Input: part model. Units: mm. Frame: model coordinates. Face numbers are marked on the shaded views. A direction names the side the tool comes from. Give positions to 0.01 mm unless a question says otherwise; leave off trailing zeros. Loops run counter-clockwise (first coordinate to the right, second up) from the corner with the lowest first, then second, coordinate; pieces in that order, holes last. Notation, with made-up numbers: M 52,-1.5 L 71,-1.5 A8 cw 71,5.5 Z; hole C 65,61.5 d11. An arc over 180 degrees is marked long. Answer as a JSON object with one key per item and string values. Group by question number.
1) First-contact query: P1, Ø2, axis at x = 0, z = -1.5, coming from the +Y side; P2, Ø1, axis at y = -3, z = -2.5, coming from the +X side; P3, Ø4, axis at x = 5.5, y = -1.5, coming from the -Z side. Flat tips, straight axial feed; report the tip coordinate or a pass-through.
2) Section query B-B on x = 6.75. Return loops of the section in (y, z), plus the area to 3 significant figures.
3) Ray query, L1, parallel to Y at x = 14, z = 1.5; L2, parallel to X at y = -3.25, z = 0.25; L3, parallel to X at y = 3, z = -2.25. Return the intervals inside material, ascending.
4) Access query for the marked faces 1 and 2. Directions: +Z, -Z, +X, -X, +Y, -Y. A direction counts if a zero-diameter tool reaches every point of the face in a straight line with its end or side. Return the directions, or none.
5) Section query A-A on x = -1. Return loops of the section in (y, z).
Autodesk Inventor part; units mm, degrees
ref_plane "Work Plane1" through (1.525, 0, 0) normal (0, 0, 1) x (1, 0, 0)
ref_plane "YZ Plane" through (0, 0, 0) normal (1, 0, 0) x (0, 1, 0)
ref_plane "XZ Plane" through (0, 0, 0) normal (0, 1, 0) x (-1, 0, 0)
sketch "Sketch1" plane through (0, 0, 0) normal (0, 0, 1) x (1, 0, 0)
  line L0 (0, 3.44) -> (0, 2.5)
  line L1 (2.4, 2.5) -> (20, 2.5)
  line L2 (20, 2.5) -> (20, 0)
  line L3 (20, 0) -> (-0.5001, 0)
  line L4 (-4.6001, 0) -> (24.1, 0)
  line L5 (-0.5001, 0) -> (-0.5001, 3.44)
  line L6 (-0.5001, 3.44) -> (0, 3.44)
  line L7 (2.4, 2.5) -> (1.9091, 2.5)
  line L8 (1.9091, 2.5) -> (0, 2.5)
  line L9 (0, -0.688) -> (0, 4.128)
  dimension "d0" = 20
  dimension "d1" = 17.6
  dimension "d2" = 5
  dimension "d9" = 0.5001
  dimension "d10" = 6.88
  dimension "d13" = 0.4909
  dimension "d14" = 5
revolve "Body" add sketch "Sketch1" angle 360 about axis through (20, 0, 0) along (-1, 0, 0)
sketch "Sketch2" plane through (-0.5001, 0, 0) normal (-1, 0, 0) x (0, 0, 1)
  line L0 (0, 4.6188) -> (4, 2.3094)
  line L1 (4, 2.3094) -> (4, -2.3094)
  line L2 (4, -2.3094) -> (0, -4.6188)
  line L3 (0, -4.6188) -> (-4, -2.3094)
  line L4 (-4, -2.3094) -> (-4, 2.3094)
  line L5 (-4, 2.3094) -> (0, 4.6188)
  point P0 (0, 0)
  point P1 (0, 0)
  dimension "d11" = 8
extrude "Head" add sketch "Sketch2" along normal blind 3
sketch "Sketch4" plane through (0, 0, 0) normal (0, 0, 1) x (1, 0, 0)
  line L0 (-3.5001, 4) -> (-3.5001, 4.6188)
  line L1 (-3.5001, 4.6188) -> (-3.1428, 4.6188)
  line L2 (-3.1428, 4.6188) -> (-3.5001, 4)
  line L3 (-4.1001, 0) -> (0.0999, 0)
  line L4 (-0.5001, 4.6188) -> (-3.5001, 4.6188)
  line L5 (-3.5001, 2.3094) -> (-3.5001, 4.6188)
  dimension "d5" = 30
  dimension "d19" = 8
revolve "Chamfer1" cut sketch "Sketch4" angle 360 about axis through (-10, 0, 0) along (1, 0, 0)
thread "Thread"
chamfer "Chamfer2" distance 0.4908 distance2 0.4909 1 edges at (20, -2.5, 0) measured on face at (20, 0.7379, -0.3873)
ref_plane "Work Plane1" through (1.525, 0, 0) normal (0, 0, 1) x (1, 0, 0)
equation "\"d0\" = NLG"
equation "\"d1\" = GEL"
equation "\"d2\" = GD"
equation "\"d10\" = SD2"
equation "\"d14\" = BDM"
equation "\"d11\" = SW"
equation "\"d3\" = KOH - SD"
equation "\"d5\" = ANG1"
equation "\"d19\" = SW0"
equation "\"d15\" = GEL"
equation "\"d6\" = -0.5 * SPD + 0.5 * GD"
equation "\"NLG\" = 20"
equation "\"GD\" = NND"
equation "\"BDM\" = NND"
equation "\"KOH\" = 3.5"
equation "\"GEL\" = 17.6"
equation "\"SW\" = 8"
equation "\"SW0\" = SW"
equation "\"SPD\" = NND - 1.2269 * PTC"
equation "\"SD2\" = 6.88"
equation "\"SD\" = 0.5"
equation "\"ANG1\" = 30deg"
equation "\"GAL\" = 0.61345 * PTC"
equation "\"GUL\" = 0.61345 * PTC"
equation "\"RR\" = 0.2"
equation "\"GD1\" = THREADDIA - 1.2269 * PTC"
equation "\"THREADDIA\" = 5"
equation "\"SDH\" = SD2"
equation "\"SDHG\" = 2.4"
equation "\"TOA\" = 30deg"
equation "\"PTC\" = 0.8"
equation "\"NND\" = 5"
equation "\"E0\" = 9.24"
properties part number "ISO 4017 - M5 x 20" material "Stainless Steel, 440C"
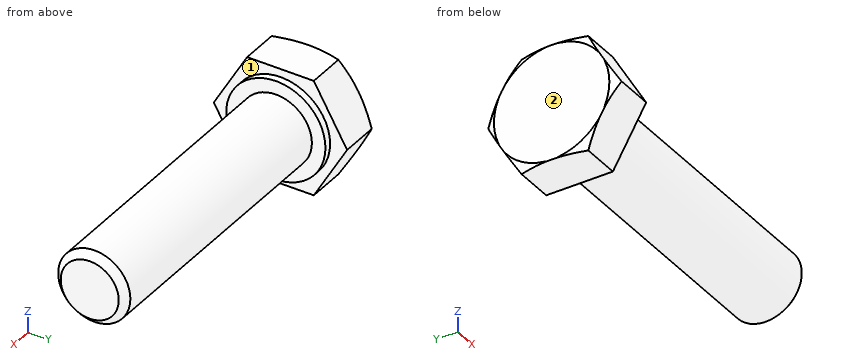
Output:
{
 "1": {"P1": "stops at y = 4.25", "P2": "stops at x = 0", "P3": "stops at z = -2.5"},
 "2": {"outline": "C 0,0 d5", "area": "19.6 mm^2"},
 "3": {"L1": "y = -2 to 2", "L2": "x = -3.5 to 0", "L3": "x = -3.5 to -0.5"},
 "4": {"face 1": "+X", "face 2": "+Z, -Z, -X, +Y, -Y"},
 "5": {"outline": "M -4.62,0 L -2.31,-4 L 2.31,-4 L 4.62,0 L 2.31,4 L -2.31,4 Z"}
}
